Autodesk Inventor part; units mm, degrees
ref_plane "YZ Plane" through (0, 0, 0) normal (1, 0, 0) x (0, 1, 0)
ref_plane "XZ Plane" through (0, 0, 0) normal (0, 1, 0) x (-1, 0, 0)
ref_plane "XY Plane" through (0, 0, 0) normal (0, 0, 1) x (1, 0, 0)
sketch "Sketch1" plane through (0, 0, 0) normal (0, 0, 1) x (1, 0, 0)
  line L0 (0, 0) -> (25.4, 0)
  line L1 (25.4, 0) -> (25.4, 25.4)
  line L2 (25.4, 25.4) -> (0, 25.4)
  line L3 (0, 25.4) -> (0, 0)
  line L4 (3.175, 22.225) -> (22.225, 22.225)
  line L5 (22.225, 22.225) -> (22.225, 3.175)
  line L6 (22.225, 3.175) -> (3.175, 3.175)
  line L7 (3.175, 3.175) -> (3.175, 22.225)
  dimension "d0" = 25.4
  dimension "d1" = 25.4
  dimension "d2" = 3.175
extrude "Extrusion1" add sketch "Sketch1" along normal blind 419.1
sketch "Sketch2" plane through (25.4, 0, 0) normal (1, 0, 0) x (0, 0, -1)
  line L0 (-419.1, 0) -> (-419.1, 25.4)
  line L1 (0, 0) -> (-419.1, 0)
  line L2 (-419.1, 12.7) -> (-400.05, 12.7) construction
  circle A0 centre (-400.05, 12.7) radius 3.302 construction
  circle A1 centre (-374.65, 12.7) radius 3.302
  circle A2 centre (-349.25, 12.7) radius 3.302
  circle A3 centre (-323.85, 12.7) radius 3.302
  circle A4 centre (-298.45, 12.7) radius 3.302
  circle A5 centre (-273.05, 12.7) radius 3.302
  circle A6 centre (-247.65, 12.7) radius 3.302
  circle A7 centre (-222.25, 12.7) radius 3.302
  circle A8 centre (-196.85, 12.7) radius 3.302
  circle A9 centre (-171.45, 12.7) radius 3.302
  circle A10 centre (-146.05, 12.7) radius 3.302
  circle A11 centre (-120.65, 12.7) radius 3.302
  circle A12 centre (-95.25, 12.7) radius 3.302
  circle A13 centre (-69.85, 12.7) radius 3.302
  circle A14 centre (-44.45, 12.7) radius 3.302
  circle A15 centre (-19.05, 12.7) radius 3.302 construction
  line L3 (0, 0) -> (0, 25.4)
  circle A16 centre (-406.4, 12.7) radius 3.302
  circle A17 centre (-12.7, 12.7) radius 3.302
  line L4 (-12.7, 12.7) -> (0, 12.7) construction
  dimension "d5" = 19.05
  dimension "d7" = 6.604
  dimension "d10" = 419.1
  dimension "d13" = 25.4
  dimension "d18" = 19.05
  dimension "d19" = 12.7
  dimension "d20" = 6.604
  dimension "d21" = 6.604
  dimension "d22" = 12.7
extrude "Extrusion2" cut sketch "Sketch2" against normal through all
sketch "Sketch3" plane through (0, 25.4, 0) normal (0, 1, 0) x (1, 0, 0)
  line L0 (25.4, 0) -> (0, 0)
  line L1 (25.4, -419.1) -> (0, -419.1)
  circle A0 centre (12.7, -400.05) radius 3.302 construction
  line L2 (12.7, -419.1) -> (12.7, 0) construction
  circle A1 centre (12.7, -374.65) radius 3.302 construction
  circle A2 centre (12.7, -349.25) radius 3.302
  circle A3 centre (12.7, -323.85) radius 3.302
  circle A4 centre (12.7, -298.45) radius 3.302
  circle A5 centre (12.7, -273.05) radius 3.302
  circle A6 centre (12.7, -247.65) radius 3.302
  circle A7 centre (12.7, -222.25) radius 3.302
  circle A8 centre (12.7, -196.85) radius 3.302
  circle A9 centre (12.7, -171.45) radius 3.302
  circle A10 centre (12.7, -146.05) radius 3.302
  circle A11 centre (12.7, -120.65) radius 3.302
  circle A12 centre (12.7, -95.25) radius 3.302
  circle A13 centre (12.7, -69.85) radius 3.302
  circle A14 centre (12.7, -44.45) radius 3.302 construction
  circle A15 centre (12.7, -19.05) radius 3.302 construction
  dimension "d23" = 6.604
  dimension "d25" = 19.05
  dimension "d28" = 25.4
  dimension "d33" = 19.05
extrude "Extrusion3" cut sketch "Sketch3" against normal blind 25.4
equation "\"d13\" = -0.133333 * d5 + 0.0666667 * d10"
equation "\"d20\" = d7"
equation "\"d21\" = d7"
equation "\"d22\" = d19"
properties part number "Chassis V1.500 Part7" material "Aluminum 6061"
The listing builds one solid part. Answer for the finished solid, in the listing's coordinates (mm). A direction names the side the tool comes from. Give positions to 0.01 mm unless a question says otherwise; leave off trailing zeros. Write each loop counter-clockwise with the first axis right and the second up, starting at its lowest first coordinate (ties: lowest second). Pieces come first, ordered by that corner, then holes.
1) A tool of negligible diameter and unlimited length cuts with its end or side. For faces 1 (the face through (13, 3.175, 207)), 2 (the face through (14.48, 23.83, 67.07)), from which of +Z, -Z, +X, -X, +Y, -Y can it reach the whole face along a straight path? Write none if from no direction.
2) For a pull along Y with two mould halves and no side action, classify faces 3 (the face through (1.6, 15.5, 118.9)), 4 (the face through (13, 25.4, 207)), 5 (the face through (1.61, 13.69, 346.1)), 6 (the face through (11.984, 1.61, 250.873)) as pulls with the +Y half, pulls with the -Y half, needs draft (parallel to the pull), parting line crosses it, or undercut.
3) Find the intervals of material crossed by L1, parallel to X at y = 19.5, z = 274 (3 decimals); L2, parallel to Y at x = 0.9, z = 273.05, in increasing order.
4) Section A-A (z = 288) is taken. Write down the section's boundary in (x, y) (3 decimals), and give its area (3 significant figures).
Response:
1. face 1: +Z, -Z
1. face 2: +Y, -Y
2. face 3: undercut
2. face 4: pulls with the +Y half
2. face 5: undercut
2. face 6: needs draft
3. L1: x = 0 to 3.175, 22.225 to 25.4
3. L2: y = 0 to 9.4, 16 to 25.4
4. outline: (0, 0) - (25.4, 0) - (25.4, 25.4) - (0, 25.4) - close; hole (3.175, 3.175) - (22.225, 3.175) - (22.225, 22.225) - (3.175, 22.225) - close
4. area: 282 mm2
